Input: dimensioned drawing with shaded views. Units: mm. Origin: part minimum x, y, z. Coordinates: 2 decimals unless noted, no trailing zeros. Loops run counter-clockwise (first coordinate to the right, second up) from the corner with the lowest first, then second, coordinate; pieces in that order, holes last. Notation, with made-up numbers: (-0.5, 57.5) - (20.5, 57.5) arc R13 cw to (20.5, 82.5) - close; hole circle Ø9 at (8.25, 34.25). An arc over 180 degrees is marked (long way). Write item = value, one per line. Start each with the question number.
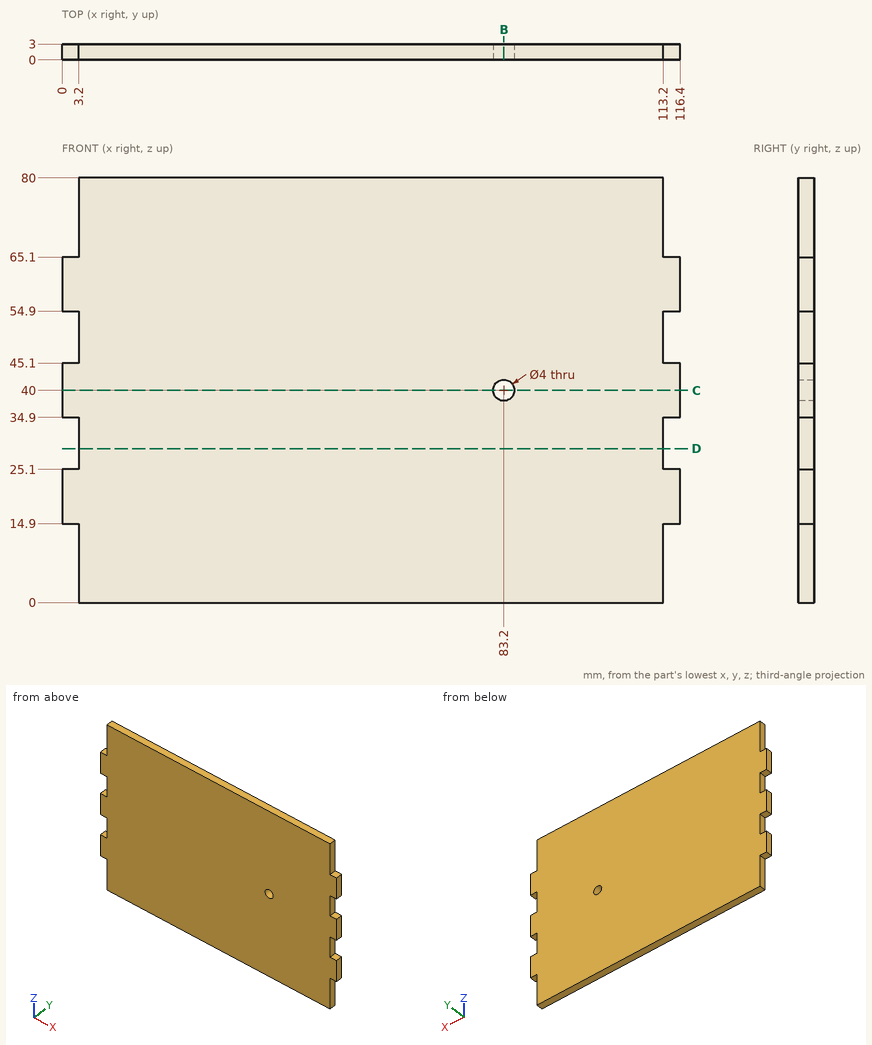
Item 1: Cut plane B-B on x = 83.2. Return loops of the section in (y, z), plus the area to 3 significant figures.
Item 2: Ray query, line 1 (X direction, y = 2.1, z = 40); line 2 (X direction, y = 0.85, z = 6.5); line 3 (Z direction, x = 82, y = 1.7). Return the intervals inside material, ascending.
Item 3: Cut plane C-C on z = 40. Return loops of the section in (x, y).
Item 4: Pin query (flat end, axial travel): pin 1 (1.5 mm diameter, centred on x = 1, y = 1, fed in from +Z); pin 2 (0.9 mm diameter, centred on y = 1.5, z = 31.5, fed in from +X); pin 3 (1.5 mm diameter, centred on x = 114.5, y = 2, fed in from -Z). Return the tip coordinate at first contact, or that it passes through.
Item 5: Cut plane D-D on z = 29. Return loops of the section in (x, y), plus the area to 3 significant figures.
Recorded:
q1.outline = (0, 0) - (3, 0) - (3, 38) - (0, 38) - close; (0, 42) - (3, 42) - (3, 80) - (0, 80) - close
q1.area = 228 mm²
q2.line_1 = 0 to 81.2, 85.2 to 116.4
q2.line_2 = 3.2 to 113.2
q2.line_3 = 0 to 38.4, 41.6 to 80
q3.outline = (0, 0) - (81.2, 0) - (81.2, 3) - (0, 3) - close; (85.2, 0) - (116.4, 0) - (116.4, 3) - (85.2, 3) - close
q4.pin_1 = 65.1
q4.pin_2 = 113.2
q4.pin_3 = 14.9
q5.outline = (3.2, 0) - (113.2, 0) - (113.2, 3) - (3.2, 3) - close
q5.area = 330 mm²
